from build123d import *

# Parameters (mm, degrees)
BOSS_EXTRUDE1_DEPTH  = 25
SHELL1_T             = -2.5
SKETCH2_R            = 1.75
CUT_EXTRUDE1_DEPTH   = 57.695792613
SKETCH3_R            = 1.215
CUT_EXTRUDE2_DEPTH   = 2.5
LPATTERN1_COUNT      = 2
LPATTERN1_PITCH      = 18
LPATTERN1_COUNT_DIR2 = 2
LPATTERN1_PITCH_DIR2 = 19.5


with BuildPart() as part:
    # Sketch1 → Boss-Extrude1 (new body)
    with BuildSketch(Plane.XY):
        with BuildLine():
            Line((0, 4), (0, 38))
            ThreePointArc((0, 38), (1.171572875, 40.828427125), (4, 42))
            Line((4, 42), (24.73, 42))
            ThreePointArc((24.73, 42), (27.558427125, 40.828427125), (28.73, 38))
            Line((28.73, 38), (28.73, 4))
            ThreePointArc((28.73, 4), (27.558427125, 1.171572875), (24.73, 0))
            Line((24.73, 0), (4, 0))
            ThreePointArc((4, 0), (1.171572875, 1.171572875), (0, 4))
        make_face()
    extrude(amount=BOSS_EXTRUDE1_DEPTH)

    # Shell1
    shell1_openings = [part.faces().sort_by_distance(p)[0] for p in [
        (14.365, 21, 25),
        (14.365, 21, 0),
    ]]
    offset(amount=SHELL1_T, openings=shell1_openings, kind=Kind.INTERSECTION)

    # Sketch2 → Cut-Extrude1 (cut, through all)
    with BuildSketch(Plane(origin=(0, 42, 0), x_dir=(1, 0, 0), z_dir=(0, 1, 0))):
        with Locations(Location((14.365, -12.5, 0), (0, 0, 270))):
            Circle(SKETCH2_R)
    extrude(amount=-CUT_EXTRUDE1_DEPTH, mode=Mode.SUBTRACT)

    # Sketch3 → Cut-Extrude2 (cut)
    with BuildSketch(Plane(origin=(28.73, 0, 0), x_dir=(0, 0, -1), z_dir=(1, 0, 0))):
        with Locations(Location((-22.25, 31.25, 0), (0, 0, 90))):
            Circle(SKETCH3_R)
    cut_extrude2 = extrude(amount=-CUT_EXTRUDE2_DEPTH, mode=Mode.SUBTRACT)

    # LPattern1: Cut-Extrude2 2 × 2
    with Locations(*[(0, -i * LPATTERN1_PITCH, -j * LPATTERN1_PITCH_DIR2) for i in range(LPATTERN1_COUNT) for j in range(LPATTERN1_COUNT_DIR2) if (i, j) != (0, 0)]):
        add(cut_extrude2, mode=Mode.SUBTRACT)


solid = part.part
For this review, take the finished solid that the model builds, in its own axes (mm). A direction names the side the tool comes from. Coordinates: 2 decimals unless noted, no trailing zeros. Order: outer loops, then holes, each group sorted by start corner. A loop starts at its lowest first (then second) coordinate and runs counter-clockwise, first axis right, second up. Notation, with made-up numbers: (-29, 13) - (29, 13) arc R10 cw to (29, 25) - close; hole circle Ø3 at (21, 73.5). An arc over 180 degrees is marked (long way). Use one line per item in the form item = value.
Q1. For P1, Ø1.9, axis at y = 13.25, z = 22.25, coming from the +X side, flat-tipped, find the tip position at first contact; note if it passes through.
Checked values:
P1 = 2.5
Q2. Draft analysis for pull direction Y (two halves, no side actions). For faces 1 (the cylindrical face through (27.498, 12.987, 21.064)), 2 (the flat face through (2, 21, 0)), 3 (the cylindrical face through (27.498, 30.286, 21.511)), 4 (the cylindrical face through (27.589, 1.203, 12.325)), state which applies: +Y half, -Y half, draft (parallel to the pull), parting line (faces both ways), or undercut.
Checked values:
face_1 = undercut
face_2 = draft
face_3 = undercut
face_4 = -Y half
Q3. Consider section B-B (y = 15). Give the boundary of the cut face in (x, z).
Checked values:
outline = (0, 0) - (2.5, 0) - (2.5, 25) - (0, 25) - close; (26.23, 0) - (28.73, 0) - (28.73, 25) - (26.23, 25) - close
Q4. Consider section A-A (x = 19). Give the boundary of the cut face in (y, z).
Checked values:
outline = (0, 0) - (2.5, 0) - (2.5, 25) - (0, 25) - close; (39.5, 0) - (42, 0) - (42, 25) - (39.5, 25) - close
Q5. Consider section D-D (z = 5.25). Give the boundary of the cut face in (x, y).
Checked values:
outline = (0, 4) arc R4 ccw to (4, 0) - (24.73, 0) arc R4 ccw to (28.73, 4) - (28.73, 38) arc R4 ccw to (24.73, 42) - (4, 42) arc R4 ccw to (0, 38) - close; hole (2.5, 4) arc R1.5 ccw to (4, 2.5) - (24.73, 2.5) arc R1.5 ccw to (26.23, 4) - (26.23, 38) arc R1.5 ccw to (24.73, 39.5) - (4, 39.5) arc R1.5 ccw to (2.5, 38) - close
Q6. Consider section C-C (z = 2.75). Give the boundary of the cut face in (x, y) (3 decimals), then the cut area to 3 significant figures.
Checked values:
outline = (0, 4) arc R4 ccw to (4, 0) - (24.73, 0) arc R4 ccw to (28.73, 4) - (28.73, 12.035) - (26.23, 12.035) - (26.23, 4) arc R1.5 cw to (24.73, 2.5) - (4, 2.5) arc R1.5 cw to (2.5, 4) - (2.5, 38) arc R1.5 cw to (4, 39.5) - (24.73, 39.5) arc R1.5 cw to (26.23, 38) - (26.23, 32.465) - (28.73, 32.465) - (28.73, 38) arc R4 ccw to (24.73, 42) - (4, 42) arc R4 ccw to (0, 38) - close; (26.23, 14.465) - (28.73, 14.465) - (28.73, 30.035) - (26.23, 30.035) - close
area = 305 mm2
Q7. For probe 1 along Z at (x, y) = (27.2, 31.25) (3 decimals); probe 2 along X at (y, z) = (37.5, 8.5); probe 3 along Y at (x, z) = (19, 22.5), list the stretches that pass through material, from the lowest coordinate up. Write a range as from..to.
Checked values:
probe_1 = 0..1.535, 3.965..21.035, 23.465..25
probe_2 = 0..2.5, 26.23..28.73
probe_3 = 0..2.5, 39.5..42
Q8. For faces 5 (the cylindrical face through (27.498, 30.036, 2.803)), 6 (the flat face through (0, 21, 12)), 7 (the flat face through (17, 39.5, 12)), list the 3-axis set-ups (+Z, -Z, +X, -X, +Y, -Y) from which the entire face can be reached by the end or side of a thin tool; tool diameter is ignored.
Checked values:
face_5 = +X
face_6 = +Z, -Z, -X, +Y, -Y
face_7 = +Z, -Z
